```python
from build123d import *

# Parameters (mm, degrees)
SKETCH_1_R             = 7
SKETCH_1_R_2           = 5.5
EXTRUDE_1_DEPTH        = 30
EXTRUDE_START          = -7
SKETCH_2_R             = 15
SKETCH_2_R_2           = 5.5
EXTRUDE_2_DEPTH        = 7
SKETCH_5_W             = 5.5
SKETCH_5_H             = 9
CUT_EXTRUDE_4_DEPTH    = 15
HOLE_WIZARD_M3_1_D     = 2.5
HOLE_WIZARD_M3_1_DEPTH = 9.5
HOLE_WIZARD_M3_1_TIP   = 0.751075774
FILLET_1_R             = 1
SKETCH1_R              = 7.5
EXTRUDE1_DEPTH         = 5
CHAMFER1_SIZE          = 1
SKETCH_9_R             = 18
CUT_EXTRUDE_1_DEPTH    = 55
SKETCH_10_R            = 9
CUT_EXTRUDE_2_DEPTH    = 22.914607001
CHAMFER_5_SIZE         = 1
SKETCH_11_R            = 2.25
CUT_EXTRUDE_3_DEPTH    = 5.5


with BuildPart() as part:
    # 草图1 → 拉伸1 (new, symmetric)
    with BuildSketch(Plane.XY):
        Circle(SKETCH_1_R)
        Circle(SKETCH_1_R_2, mode=Mode.SUBTRACT)
    extrude(amount=EXTRUDE_1_DEPTH, both=True)

    # 草图2 → 拉伸2 (add)
    with BuildSketch(Plane.XY.offset(30).offset(EXTRUDE_START)):
        Circle(SKETCH_2_R)
        Circle(SKETCH_2_R_2, mode=Mode.SUBTRACT)
    extrude_2 = extrude(amount=EXTRUDE_2_DEPTH)

    # 镜向1: 拉伸2 across plane
    add(extrude_2.mirror(Plane.XY))

    # 草图5 → 拉伸4 (cut, symmetric)
    with BuildSketch(Plane(origin=(0, 0, 0), x_dir=(0, 0, -1), z_dir=(1, 0, 0))):
        with Locations((-27.25, -15.5)):
            Rectangle(SKETCH_5_W, SKETCH_5_H)
        with Locations((27.25, -15.5)):
            Rectangle(SKETCH_5_W, SKETCH_5_H)
    extrude(amount=CUT_EXTRUDE_4_DEPTH, both=True, mode=Mode.SUBTRACT)

    # M3 螺纹孔1
    with Locations(Plane(origin=(-8, -11, 27.5), x_dir=(0, 0, -1), z_dir=(0, -1, 0))):
        with Locations((0, 0), (0, 16), (55, 0), (55, 16)):
            Hole(HOLE_WIZARD_M3_1_D / 2, depth=HOLE_WIZARD_M3_1_DEPTH)
            with Locations((0, 0, -(HOLE_WIZARD_M3_1_DEPTH + HOLE_WIZARD_M3_1_TIP / 2))):  # 118° drill point
                Cone(0, HOLE_WIZARD_M3_1_D / 2, HOLE_WIZARD_M3_1_TIP, mode=Mode.SUBTRACT)

    # 圆角1
    fillet_1_edges = [part.edges().sort_by_distance(p)[0] for p in [
        (-7, 0, -23),
        (-7, 0, 23),
    ]]
    fillet(fillet_1_edges, radius=FILLET_1_R)

    # Sketch1 → Extrude1 (cut)
    with BuildSketch(Plane(origin=(0, 0, 30), x_dir=(-1, 0, 0), z_dir=(0, 0, -1))):
        Circle(SKETCH1_R)
    extrude(amount=EXTRUDE1_DEPTH, mode=Mode.SUBTRACT)

    # Chamfer1
    chamfer1_edges = [part.edges().sort_by_distance(p)[0] for p in [
        (-5.5, 0, 25),
    ]]
    chamfer(chamfer1_edges, length=CHAMFER1_SIZE)

    # 草图9 → 切除-拉伸1 (cut)
    with BuildSketch(Plane(origin=(0, 0, -24.5), x_dir=(-1, 0, 0), z_dir=(0, 0, -1))):
        Circle(SKETCH_9_R)
    extrude(amount=-CUT_EXTRUDE_1_DEPTH, mode=Mode.SUBTRACT)

    # 草图10 → 切除-拉伸2 (cut, through all)
    with BuildSketch(Plane(origin=(0, 0, -30), x_dir=(-1, 0, 0), z_dir=(0, 0, -1))):
        Circle(SKETCH_10_R)
    extrude(amount=-CUT_EXTRUDE_2_DEPTH, mode=Mode.SUBTRACT)

    # 倒角5
    chamfer_5_edges = [part.edges().sort_by_distance(p)[0] for p in [
        (0, 15, -30),
        (0, 15, -24.5),
    ]]
    chamfer(chamfer_5_edges, length=CHAMFER_5_SIZE)

    # 草图11 → 切除-拉伸3 (cut)
    with BuildSketch(Plane.XY.offset(-24.5)):
        with Locations(Location((0, 12, 0), (0, 0, 60.367309199))):
            Circle(SKETCH_11_R)
    extrude(amount=-CUT_EXTRUDE_3_DEPTH, mode=Mode.SUBTRACT)


solid = part.part
```
Check sheet for the modelled part. Datum: model origin and axes. Units: mm. A direction names the side the tool comes from. Coordinates: 2 decimals unless noted, no trailing zeros. Order: outer loops, then holes, each group sorted by start corner. A loop starts at its lowest first (then second) coordinate and runs counter-clockwise, first axis right, second up. Notation, with made-up numbers: (7, 38) -> (58, 38) arc R18 ccw to (58, 59) -> close; hole circle Ø9 at (-5.75, 75). An arc over 180 degrees is marked (long way). Write item = value, one per line. Start each with the question number.
1) Material ranges on L1, parallel to X at y = 12, z = -26.4; L2, parallel to Y at x = 0, z = -26.45; L3, parallel to Y at x = 2, z = -25.9, recorded low to high.
2) Cross-section at B-B (x = -8). State how many separate pieces and enclosed holes the cut face has, then the cut area to 3 significant figures.
3) Cross-section at A-A (y = 0). Enter the section's corners in (x, z).
4) Mould release check, pull along Z, two halves, no side actions. Record for faces 1 (the cylindrical face through (9.24, -7.24, -27.66)), 2 (the cylindrical face through (0.5, 14.99, -27.23)), 3 (the conical face through (-0.5, 14.39, -29.6)): +Z half, -Z half, draft (parallel to the pull), parting line (faces both ways), or undercut.
5) Go/stop test with flat-tipped pins: P1, Ø8, axis at x = 0.5, y = 2, coming from the -Z side; P2, Ø2, axis at x = -8, z = -27.5, coming from the +Y side; P3, Ø3, axis at x = 8, z = -27.5, coming from the -Y side; P4, Ø1, axis at y = -2.5, z = -27, coming from the +X side. Record where each tip stops, or that it passes through.
6) Cross-section at C-C (z = -25.1). Enter the section's corners in (x, y), then the cut area to 3 significant figures.
7) Access from +Z, -Z, +X, -X, +Y, -Y to the whole of each face (thin tool, end or side, straight path). Record for faces 4 (the cylindrical face through (-9.22, -7.24, -27.77)), 5 (the flat face through (0, -11, -27)).
Ans:
q1.L1 = -9 to -2.25, 2.25 to 9
q1.L2 = -11 to -9, 9 to 9.75, 14.25 to 15
q1.L3 = -11 to -8.77, 8.77 to 10.97, 13.03 to 14.87
q2.separate_pieces = 3
q2.enclosed_holes = 0
q2.area = 66.5 mm²
q3.outline = (-15, -29) -> (-14, -30) -> (-9, -30) -> (-9, -24.5) -> (-14, -24.5) -> (-15, -25.5) -> close; (9, -30) -> (14, -30) -> (15, -29) -> (15, -25.5) -> (14, -24.5) -> (9, -24.5) -> close
q4.face_1 = undercut
q4.face_2 = draft
q4.face_3 = -Z half
q5.P1 = through
q5.P2 = 13.27
q5.P3 = -11
q5.P4 = 14.87
q6.outline = (-9.6, -11) -> (9.6, -11) arc R14.6 ccw (long way) to start; hole circle Ø18 at (0, 0); hole circle Ø4.5 at (0, 12)
q6.area = 352 mm²
q7.face_4 = -Y
q7.face_5 = +Z, -Z, +X, -X, -Y
